Here's how the part is built. I have some questions about the finished solid (model axes, mm). A direction names the side the tool comes from. Round coordinates to 2 decimals unless told otherwise and drop trailing zeros. Write each loop counter-clockwise with the first axis right and the second up, starting at its lowest first coordinate (ties: lowest second). Pieces come first, ordered by that corner, then holes. Notation, with made-up numbers: (82.25, -17) -> (110.25, -17) arc R14 ccw to (110.25, -3) -> close; hole circle Ø4 at (-0.5, -27). An arc over 180 degrees is marked (long way). Put each result on its own line as item: value. Start each with the question number.
1. Which directions (+Z, -Z, +X, -X, +Y, -Y) give clear straight access to the entire face, cutting with the end or side of a thin tool? Please do faces 4 (the face through (8.63, 2.028, -3.806)), 5 (the face through (-7, 4, 6)).
2. For pin 1 (2.5 mm diameter, centred on x = -24.31, y = 44, fed in from -Z); pin 2 (10 mm diameter, centred on x = -22.5, z = 21, fed in from +Y); pin 3 (5.5 mm diameter, centred on x = 11.69, y = 44, fed in from -Z); pin 4 (2 mm diameter, centred on x = 15, z = 13, fed in from +Y), each with a flat end and sliding along its axis, tell me the tip position at first contact or that it passes through.
3. Suppose I cut it at D-D (y = 29). Please give me the cut outline in (x, z), then the cut area to 3 significant figures.
4. Suppose I cut it at C-C (x = -19.5). Please give me the cut outline in (y, z), then the cut area to 3 significant figures.
5. Suppose I cut it at B-B (z = 27.5). Please give me the cut outline in (x, y), then the cut area to 3 significant figures.
6. I need wall thicknesses on probe 1 along Z at (x, y) = (11.5, 2.5); probe 2 along Z at (x, y) = (6.5, 45); probe 3 along Y at (x, z) = (-28, 4). Which ranges of each line are inside material? Lowest first, please. Write a range as from..to.
7. Suppose I cut it at A-A (y = 14). Please give me the cut outline in (x, z), then the cut area to 3 significant figures.
8. We'd pull the mould along Z, two halves only. Please class faces 1 (the face through (8.63, 2.028, 14.394)), 2 (the face through (-7, 2, -12.791)), 3 (the face through (-34.312, 18.9, 25.4)): +Z half, -Z half, draft (parallel to the pull), parting line (faces both ways), or undercut.
```python
from build123d import *

# Parameters (mm, degrees)
SKETCH_2_W          = 56
SKETCH_2_H          = 4
EXTRUDE_1_DEPTH     = 54
SKETCH_2_3_W        = 56
SKETCH_2_3_H        = 38
EXTRUDE_2_DEPTH     = 4
SKETCH_3_R          = 2.15
CUT_EXTRUDE_1_DEPTH = 4
SKETCH_4_R          = 1.7
SKETCH_4_R_2        = 7.2
CUT_EXTRUDE_3_DEPTH = 10


with BuildPart() as part:
    # Sketch 2 → Extrude 1 (new body)
    with BuildSketch(Plane(origin=(0, 0, 0), x_dir=(1, 0, 0), z_dir=(0, 1, 0))):
        with Locations((-6.312292359, -27.209302326)):
            Rectangle(SKETCH_2_W, SKETCH_2_H)
    extrude(amount=EXTRUDE_1_DEPTH)

    # Sketch 2_3 → Extrude 2 (add)
    with BuildSketch(Plane(origin=(0, 0, 0), x_dir=(1, 0, 0), z_dir=(0, 1, 0))):
        with Locations((-6.312292359, -6.209302326)):
            Rectangle(SKETCH_2_3_W, SKETCH_2_3_H)
    extrude(amount=EXTRUDE_2_DEPTH)

    # Sketch 3 → Cut-Extrude 1 (cut)
    with BuildSketch(Plane(origin=(0, 0, 25.209302326), x_dir=(-1, 0, 0), z_dir=(0, 0, -1))):
        with Locations((-11.687707641, 14)):
            Circle(SKETCH_3_R)
        with Locations((-11.687707641, 44)):
            Circle(SKETCH_3_R)
        with Locations(Location((24.312292359, 44, 0), (0, 0, 180))):
            Circle(SKETCH_3_R)
        with Locations((24.312292359, 14)):
            Circle(SKETCH_3_R)
        with Locations((6.312292359, 29)):
            Circle(SKETCH_3_R)
    extrude(amount=-CUT_EXTRUDE_1_DEPTH, mode=Mode.SUBTRACT)

    # Sketch 4 → Cut-Extrude 3 (cut)
    with BuildSketch(Plane(origin=(0, 4, 0), x_dir=(1, 0, 0), z_dir=(0, 1, 0))):
        with Locations(Location((-22.762292359, -13.609302326, 0), (0, 0, 270))):
            Circle(SKETCH_4_R)
        with Locations(Location((-22.762292359, 4.590697674, 0), (0, 0, 270))):
            Circle(SKETCH_4_R)
        with Locations(Location((-14.512292359, -4.509302326, 0), (0, 0, 270))):
            Circle(SKETCH_4_R_2)
        with Locations(Location((10.137707641, 4.590697674, 0), (0, 0, 270))):
            Circle(SKETCH_4_R)
        with Locations(Location((10.137707641, -13.609302326, 0), (0, 0, 270))):
            Circle(SKETCH_4_R)
    extrude(amount=-CUT_EXTRUDE_3_DEPTH, mode=Mode.SUBTRACT)


solid = part.part
```
Verdict:
1. face 4: +Y, -Y
1. face 5: -Z, +X, -X, +Y
2. pin 1: passes through
2. pin 2: stops at y = 54
2. pin 3: stops at z = 25.21
2. pin 4: stops at y = 4
3. outline: (-34.31, 25.21) -> (-8.46, 25.21) -> (-8.46, 29.21) -> (-34.31, 29.21) -> close; (-4.16, 25.21) -> (21.69, 25.21) -> (21.69, 29.21) -> (-4.16, 29.21) -> close
3. area: 207 mm^2
4. outline: (0, -12.79) -> (4, -12.79) -> (4, -0.68) -> (0, -0.68) -> close; (0, 9.7) -> (4, 9.7) -> (4, 25.21) -> (54, 25.21) -> (54, 29.21) -> (0, 29.21) -> close
4. area: 326 mm^2
5. outline: (-34.31, 0) -> (21.69, 0) -> (21.69, 54) -> (-34.31, 54) -> close; hole circle Ø4.3 at (-24.31, 14); hole circle Ø4.3 at (-24.31, 44); hole circle Ø4.3 at (-6.31, 29); hole circle Ø4.3 at (11.69, 14); hole circle Ø4.3 at (11.69, 44)
5. area: 2,950 mm^2
6. probe 1: z = -12.79..-5.61, -3.57..12.59, 14.63..29.21
6. probe 2: z = 25.21..29.21
6. probe 3: y = 0..4
7. outline: (-34.31, 25.21) -> (-26.46, 25.21) -> (-26.46, 29.21) -> (-34.31, 29.21) -> close; (-22.16, 25.21) -> (9.54, 25.21) -> (9.54, 29.21) -> (-22.16, 29.21) -> close; (13.84, 25.21) -> (21.69, 25.21) -> (21.69, 29.21) -> (13.84, 29.21) -> close
7. area: 190 mm^2
8. face 1: undercut
8. face 2: -Z half
8. face 3: draft
